```python
from build123d import *

# Parameters (mm, degrees)
SKETCH1_R           = 28.399999969
BOSS_EXTRUDE1_DEPTH = 6
SKETCH2_R           = 12
BOSS_EXTRUDE2_DEPTH = 20.4
SKETCH3_R           = 3
CUT_EXTRUDE1_DEPTH  = 49.063291569
SKETCH4_R           = 2.6
CUT_EXTRUDE2_DEPTH  = 46.047530415
SKETCH6_R           = 1.65
CUT_EXTRUDE3_DEPTH  = 49.063291569


with BuildPart() as part:
    # Sketch1 → Boss-Extrude1 (new body)
    with BuildSketch(Plane(origin=(0, 0, 0), x_dir=(1, 0, 0), z_dir=(0, 1, 0))):
        with Locations(Location((0, 0, 0), (0, 0, 270))):
            Circle(SKETCH1_R)
    extrude(amount=BOSS_EXTRUDE1_DEPTH)

    # Sketch2 → Boss-Extrude2 (add)
    with BuildSketch(Plane(origin=(0, 6, 0), x_dir=(1, 0, 0), z_dir=(0, 1, 0))):
        with Locations(Location((0, 0, 0), (0, 0, 270))):
            Circle(SKETCH2_R)
    extrude(amount=BOSS_EXTRUDE2_DEPTH)

    # Sketch3 → Cut-Extrude1 (cut, through all)
    with BuildSketch(Plane(origin=(0, 26.4, 0), x_dir=(1, 0, 0), z_dir=(0, 1, 0))):
        with Locations(Location((0, 0, 0), (0, 0, 270))):
            Circle(SKETCH3_R)
    extrude(amount=-CUT_EXTRUDE1_DEPTH, mode=Mode.SUBTRACT)

    # Sketch4 → Cut-Extrude2 (cut, through all)
    with BuildSketch(Plane(origin=(0, 6, 0), x_dir=(1, 0, 0), z_dir=(0, 1, 0))):
        with Locations(Location((23.75, 0, 0), (0, 0, 270))):
            Circle(SKETCH4_R)
        with Locations(Location((11.875, -20.56810334, 0), (0, 0, 270))):
            Circle(SKETCH4_R)
        with Locations(Location((-11.875, -20.56810334, 0), (0, 0, 270))):
            Circle(SKETCH4_R)
        with Locations(Location((-23.75, 0, 0), (0, 0, 270))):
            Circle(SKETCH4_R)
        with Locations(Location((-11.875, 20.56810334, 0), (0, 0, 270))):
            Circle(SKETCH4_R)
        with Locations(Location((11.875, 20.56810334, 0), (0, 0, 270))):
            Circle(SKETCH4_R)
    extrude(amount=-CUT_EXTRUDE2_DEPTH, mode=Mode.SUBTRACT)

    # Sketch6 → Cut-Extrude3 (cut, through all)
    with BuildSketch(Plane(origin=(0, 0, 0), x_dir=(0, 0, -1), z_dir=(1, 0, 0))):
        with Locations((0, 16.2)):
            Circle(SKETCH6_R)
    extrude(amount=-CUT_EXTRUDE3_DEPTH, mode=Mode.SUBTRACT)


solid = part.part
```
Input: part model. Units: mm. Frame: model coordinates. A direction names the side the tool comes from. Round coordinates to 2 decimals unless told otherwise and drop trailing zeros. Loops run counter-clockwise (first coordinate to the right, second up) from the corner with the lowest first, then second, coordinate; pieces in that order, holes last. Notation, with made-up numbers: (-9, 39.25) -> (37, 39.25) arc R12 ccw to (37, 50.25) -> close; hole circle Ø5 at (82.5, 16.5). An arc over 180 degrees is marked (long way). Write each question's results on one line, items separated by ' | '.
1. Mould query, pull axis Y, two halves, no side actions, for faces 1 (the face through (-12.2, 6, -0.4)), 2 (the face through (-7.188, 15.568, -1.524)), 3 (the face through (10.879, 3.042, -18.166)). Classes: +Y half, -Y half, draft (parallel to the pull), parting line (faces both ways), or undercut.
Geometry results:
face 1: +Y half | face 2: undercut | face 3: draft
2. Section A-A (x = 0). Return loops of the section in (y, z), and give its area (3 significant figures).
Geometry results:
outline: (0, -28.4) -> (6, -28.4) -> (6, -12) -> (26.4, -12) -> (26.4, -3) -> (0, -3) -> close; (0, 3) -> (26.4, 3) -> (26.4, 12) -> (6, 12) -> (6, 28.4) -> (0, 28.4) -> close | area: 672 mm2
3. Section D-D (x = -8). Return loops of the section in (y, z), and give its area (3 significant figures).
Geometry results:
outline: (0, -27.25) -> (6, -27.25) -> (6, -8.94) -> (26.4, -8.94) -> (26.4, 8.94) -> (6, 8.94) -> (6, 27.25) -> (0, 27.25) -> close; hole circle Ø3.3 at (16.2, 0) | area: 683 mm2
4. Section C-C (y = 11.75). Return loops of the section in (x, z), and give its area (3 significant figures).
Geometry results:
outline: circle Ø24 at (0, 0); hole circle Ø6 at (0, 0) | area: 424 mm2
5. First-contact query: P1, Ø4, axis at y = 17.5, z = -3, coming from the +X side; P2, Ø7, axis at x = 11.88, z = 20.57, coming from the +Y side; P3, Ø5, axis at x = -1.5, y = 13, coming from the -Z side. Flat tips, straight axial feed; report the tip coordinate or a pass-through.
Geometry results:
P1: x = 11.96 | P2: y = 6 | P3: z = -12
6. Ray query, line 1 (X direction, y = 4.15, z = 0); line 2 (Y direction, x = 15, z = -22); line 3 (Y direction, x = -8.5, z = -0.5). Return the intervals inside material, ascending. Write a range as from..to.
Geometry results:
line 1: -28.4..-26.35, -21.15..-3, 3..21.15, 26.35..28.4 | line 2: 0..6 | line 3: 0..14.63, 17.77..26.4
7. Section B-B (z = 0). Return loops of the section in (x, y), and give its area (3 significant figures).
Geometry results:
outline: (-28.4, 0) -> (-26.35, 0) -> (-26.35, 6) -> (-28.4, 6) -> close; (-21.15, 0) -> (-3, 0) -> (-3, 14.55) -> (-12, 14.55) -> (-12, 6) -> (-21.15, 6) -> close; (-12, 17.85) -> (-3, 17.85) -> (-3, 26.4) -> (-12, 26.4) -> close; (3, 0) -> (21.15, 0) -> (21.15, 6) -> (12, 6) -> (12, 26.4) -> (3, 26.4) -> close; (26.35, 0) -> (28.4, 0) -> (28.4, 6) -> (26.35, 6) -> close | area: 580 mm2
8. Set-up query: faces 4 (the face through (-12.871, 3.042, -18.166)), 5 (the face through (3.604, 16.057, 11.446)). Return all of +Z, -Z, +X, -X, +Y, -Y with unobstructed straight access to the full face (end or side cutting, diameter ignored); none if empty.
Geometry results:
face 4: +Y, -Y | face 5: +Y
